Input: part model. Units: mm. Frame: model coordinates. A direction names the side the tool comes from. Coordinates: 2 decimals unless noted, no trailing zeros. Order: outer loops, then holes, each group sorted by start corner. A loop starts at its lowest first (then second) coordinate and runs counter-clockwise, first axis right, second up.
from build123d import *

# Parameters (mm, degrees)
F1_DEPTH = 35
F2_DEPTH = 45
F3_DEPTH = 3
F4_R     = 2


with BuildPart() as f1:
    # F0 (on Top) → F1 (new body)
    with BuildSketch(Plane.XY):
        Polygon((50, 0), (0, 0), (0, -50), (25, -50), (28, -50), (50, -50), (50, -28), (50, -25), align=None)
    extrude(amount=F1_DEPTH)

    # F0 (on Top) → F2 (join)
    with BuildSketch(Plane.XY):
        Polygon((28, -50), (25, -50), (25, -66), (28, -66), (28, -53), align=None)
        Polygon((66, -25), (50, -25), (50, -28), (53, -28), (66, -28), align=None)
        Polygon((53, -28), (50, -28), (50, -50), (28, -50), (28, -53), (53, -53), align=None)
    extrude(amount=F2_DEPTH)

    # F0 (on Top) → F3 (join)
    with BuildSketch(Plane.XY):
        Polygon((50, 0), (0, 0), (0, -50), (25, -50), (28, -50), (50, -50), (50, -28), (50, -25), align=None)
        Polygon((66, -25), (50, -25), (50, -28), (53, -28), (66, -28), align=None)
        Polygon((28, -50), (25, -50), (25, -66), (28, -66), (28, -53), align=None)
        Polygon((66, -28), (53, -28), (53, -53), (28, -53), (28, -66), (66, -66), align=None)
    extrude(amount=F3_DEPTH)

    # F4
    f4_edges = [f1.edges().sort_by_distance(p)[0] for p in [
        (47, -66, 3),
        (66, -47, 3),
        (66, -66, 1.5),
        (53, -53, 24),
        (40.5, -53, 45),
        (28, -59.5, 45),
        (53, -40.5, 45),
        (59.5, -28, 45),
        (66, -28, 24),
        (28, -66, 24),
    ]]
    fillet(f4_edges, radius=F4_R)


solid = f1.part
Item 1: Cut plane C-C on z = 38. Return loops of the section in (x, y).
Response values:
outline: (25, -66) - (26, -66) arc R2 ccw to (28, -64) - (28, -53) - (51, -53) arc R2 ccw to (53, -51) - (53, -28) - (64, -28) arc R2 ccw to (66, -26) - (66, -25) - (50, -25) - (50, -50) - (25, -50) - close
Item 2: Access query for faces 1 (the face through (0, -25, 17)), 2 (the face through (58, -28, 23)), 3 (the face through (58, -25, 22)), 4 (the face through (38, -50, 40)), 5 (the face through (25, 0, 17)). Directions: +Z, -Z, +X, -X, +Y, -Y. A direction counts if a zero-diameter tool reaches every point of the face in a straight line with its end or side. Return the directions, or none.
Response values:
face 1: +Z, -Z, -X, +Y, -Y
face 2: +Z, +X, -Y
face 3: +Z, -Z, +X, +Y
face 4: +Z, -X, +Y
face 5: +Z, -Z, +X, -X, +Y
Item 3: Cut plane D-D on x = 43. Return loops of the section in (y, z).
Response values:
outline: (-66, 0) - (0, 0) - (0, 35) - (-50, 35) - (-50, 45) - (-51, 45) arc R2 ccw to (-53, 43) - (-53, 3) - (-64, 3) arc R2 ccw to (-66, 1) - close
Item 4: Cut plane A-A on y = -38. Return loops of the section in (x, z).
Response values:
outline: (0, 0) - (66, 0) - (66, 1) arc R2 ccw to (64, 3) - (53, 3) - (53, 43) arc R2 ccw to (51, 45) - (50, 45) - (50, 35) - (0, 35) - close
Item 5: Ray query, probe 1 along X at (y, z) = (-36.5, 5.5); probe 2 along X at (y, z) = (-16, 14); probe 3 along Z at (x, y) = (22, -34.5). Return the intervals inside material, ascending.
Response values:
probe 1: x = 0 to 53
probe 2: x = 0 to 50
probe 3: z = 0 to 35
Item 6: Cut plane B-B on x = 55. Return loops of the section in (y, z).
Response values:
outline: (-66, 0) - (-25, 0) - (-25, 45) - (-26, 45) arc R2 ccw to (-28, 43) - (-28, 3) - (-64, 3) arc R2 ccw to (-66, 1) - close
Item 7: Pin query (flat end, axial travel): pin 1 Ø12 at (x, y) = (42, -42) entering from +Z; pin 2 Ø11 at (y, z) = (-36, 42.5) entering from -X; pin 3 Ø9 at (x, z) = (59.5, 14.5) entering from -Y. Return the tip coordinate at first contact, or that it passes through.
Response values:
pin 1: stops at z = 35
pin 2: stops at x = 50
pin 3: stops at y = -28
